```python
from build123d import *

# Parameters (mm, degrees)
SKETCH1_W           = 40.5
SKETCH1_H           = 37.5
PCB_DEPTH           = 1.64
FILLET1_R           = 2
MOUNT_HOLE_REACH    = 29.646
SKETCH2_R           = 1.45
SLOT_REACH          = 29.646
CUT_EXTRUDE3_REACH  = 29.646
SKETCH4_R           = 0.5
SKETCH5_W           = 34.6
SKETCH5_H           = 22.7
OLED_GLASS_DEPTH    = 1.6
SKETCH6_W           = 12
SKETCH6_H           = 3.8
BOSS_EXTRUDE3_DEPTH = 1
FILLET2_R           = 1


with BuildPart() as part:
    # Sketch1 → PCB (new body)
    with BuildSketch(Plane.XY):
        Rectangle(SKETCH1_W, SKETCH1_H)
    extrude(amount=PCB_DEPTH)

    # Fillet1
    fillet1_edges = [part.edges().sort_by_distance(p)[0] for p in [
        (-20.25, 18.75, 0.82),
        (20.25, 18.75, 0.82),
        (20.25, -18.75, 0.82),
        (-20.25, -18.75, 0.82),
    ]]
    fillet(fillet1_edges, radius=FILLET1_R)

    # Sketch2 → mount hole (cut, up to next)
    with BuildSketch(Plane.XY.offset(1.64), mode=Mode.PRIVATE) as mount_hole_sk1:
        with Locations((-17.75, 16.25)):
            Circle(SKETCH2_R)
    mount_hole_tool1 = extrude(mount_hole_sk1.sketch, amount=-MOUNT_HOLE_REACH, mode=Mode.PRIVATE) & part.part
    # Sketch2 → mount hole (cut, up to next)
    with BuildSketch(Plane.XY.offset(1.64), mode=Mode.PRIVATE) as mount_hole_sk2:
        with Locations((17.75, 16.25)):
            Circle(SKETCH2_R)
    mount_hole_tool2 = extrude(mount_hole_sk2.sketch, amount=-MOUNT_HOLE_REACH, mode=Mode.PRIVATE) & part.part
    # Sketch2 → mount hole (cut, up to next)
    with BuildSketch(Plane.XY.offset(1.64), mode=Mode.PRIVATE) as mount_hole_sk3:
        with Locations((17.75, -16.25)):
            Circle(SKETCH2_R)
    mount_hole_tool3 = extrude(mount_hole_sk3.sketch, amount=-MOUNT_HOLE_REACH, mode=Mode.PRIVATE) & part.part
    # Sketch2 → mount hole (cut, up to next)
    with BuildSketch(Plane.XY.offset(1.64), mode=Mode.PRIVATE) as mount_hole_sk4:
        with Locations((-17.75, -16.25)):
            Circle(SKETCH2_R)
    mount_hole_tool4 = extrude(mount_hole_sk4.sketch, amount=-MOUNT_HOLE_REACH, mode=Mode.PRIVATE) & part.part
    add(mount_hole_tool1.solids().sort_by_distance((-17.75, 16.25, 1.64))[0], mode=Mode.SUBTRACT)
    add(mount_hole_tool2.solids().sort_by_distance((17.75, 16.25, 1.64))[0], mode=Mode.SUBTRACT)
    add(mount_hole_tool3.solids().sort_by_distance((17.75, -16.25, 1.64))[0], mode=Mode.SUBTRACT)
    add(mount_hole_tool4.solids().sort_by_distance((-17.75, -16.25, 1.64))[0], mode=Mode.SUBTRACT)

    # Sketch3 → slot (cut, up to next)
    with BuildSketch(Plane.XY.offset(1.64), mode=Mode.PRIVATE) as slot_sk1:
        with BuildLine():
            Line((-9.4, -15.15), (9.4, -15.15))
            ThreePointArc((9.4, -15.15), (10, -15.75), (9.4, -16.35))
            Line((9.4, -16.35), (-9.4, -16.35))
            ThreePointArc((-9.4, -16.35), (-10, -15.75), (-9.4, -15.15))
        make_face()
    slot_tool1 = extrude(slot_sk1.sketch, amount=-SLOT_REACH, mode=Mode.PRIVATE) & part.part
    add(slot_tool1.solids().sort_by_distance((0, -15.75, 1.64))[0], mode=Mode.SUBTRACT)

    # Sketch4 → Cut-Extrude3 (cut, up to next)
    with BuildSketch(Plane.XY.offset(1.64), mode=Mode.PRIVATE) as cut_extrude3_sk1:
        with Locations((-8.89, 15.55)):
            Circle(SKETCH4_R)
    cut_extrude3_tool1 = extrude(cut_extrude3_sk1.sketch, amount=-CUT_EXTRUDE3_REACH, mode=Mode.PRIVATE) & part.part
    # Sketch4 → Cut-Extrude3 (cut, up to next)
    with BuildSketch(Plane.XY.offset(1.64), mode=Mode.PRIVATE) as cut_extrude3_sk2:
        with Locations((-6.35, 15.55)):
            Circle(SKETCH4_R)
    cut_extrude3_tool2 = extrude(cut_extrude3_sk2.sketch, amount=-CUT_EXTRUDE3_REACH, mode=Mode.PRIVATE) & part.part
    # Sketch4 → Cut-Extrude3 (cut, up to next)
    with BuildSketch(Plane.XY.offset(1.64), mode=Mode.PRIVATE) as cut_extrude3_sk3:
        with Locations((-3.81, 15.55)):
            Circle(SKETCH4_R)
    cut_extrude3_tool3 = extrude(cut_extrude3_sk3.sketch, amount=-CUT_EXTRUDE3_REACH, mode=Mode.PRIVATE) & part.part
    # Sketch4 → Cut-Extrude3 (cut, up to next)
    with BuildSketch(Plane.XY.offset(1.64), mode=Mode.PRIVATE) as cut_extrude3_sk4:
        with Locations((-1.27, 15.55)):
            Circle(SKETCH4_R)
    cut_extrude3_tool4 = extrude(cut_extrude3_sk4.sketch, amount=-CUT_EXTRUDE3_REACH, mode=Mode.PRIVATE) & part.part
    # Sketch4 → Cut-Extrude3 (cut, up to next)
    with BuildSketch(Plane.XY.offset(1.64), mode=Mode.PRIVATE) as cut_extrude3_sk5:
        with Locations((1.27, 15.55)):
            Circle(SKETCH4_R)
    cut_extrude3_tool5 = extrude(cut_extrude3_sk5.sketch, amount=-CUT_EXTRUDE3_REACH, mode=Mode.PRIVATE) & part.part
    # Sketch4 → Cut-Extrude3 (cut, up to next)
    with BuildSketch(Plane.XY.offset(1.64), mode=Mode.PRIVATE) as cut_extrude3_sk6:
        with Locations((3.81, 15.55)):
            Circle(SKETCH4_R)
    cut_extrude3_tool6 = extrude(cut_extrude3_sk6.sketch, amount=-CUT_EXTRUDE3_REACH, mode=Mode.PRIVATE) & part.part
    # Sketch4 → Cut-Extrude3 (cut, up to next)
    with BuildSketch(Plane.XY.offset(1.64), mode=Mode.PRIVATE) as cut_extrude3_sk7:
        with Locations((6.35, 15.55)):
            Circle(SKETCH4_R)
    cut_extrude3_tool7 = extrude(cut_extrude3_sk7.sketch, amount=-CUT_EXTRUDE3_REACH, mode=Mode.PRIVATE) & part.part
    # Sketch4 → Cut-Extrude3 (cut, up to next)
    with BuildSketch(Plane.XY.offset(1.64), mode=Mode.PRIVATE) as cut_extrude3_sk8:
        with Locations((8.89, 15.55)):
            Circle(SKETCH4_R)
    cut_extrude3_tool8 = extrude(cut_extrude3_sk8.sketch, amount=-CUT_EXTRUDE3_REACH, mode=Mode.PRIVATE) & part.part
    add(cut_extrude3_tool1.solids().sort_by_distance((-8.89, 15.55, 1.64))[0], mode=Mode.SUBTRACT)
    add(cut_extrude3_tool2.solids().sort_by_distance((-6.35, 15.55, 1.64))[0], mode=Mode.SUBTRACT)
    add(cut_extrude3_tool3.solids().sort_by_distance((-3.81, 15.55, 1.64))[0], mode=Mode.SUBTRACT)
    add(cut_extrude3_tool4.solids().sort_by_distance((-1.27, 15.55, 1.64))[0], mode=Mode.SUBTRACT)
    add(cut_extrude3_tool5.solids().sort_by_distance((1.27, 15.55, 1.64))[0], mode=Mode.SUBTRACT)
    add(cut_extrude3_tool6.solids().sort_by_distance((3.81, 15.55, 1.64))[0], mode=Mode.SUBTRACT)
    add(cut_extrude3_tool7.solids().sort_by_distance((6.35, 15.55, 1.64))[0], mode=Mode.SUBTRACT)
    add(cut_extrude3_tool8.solids().sort_by_distance((8.89, 15.55, 1.64))[0], mode=Mode.SUBTRACT)

    # Sketch5 → OLED glass (add)
    with BuildSketch(Plane.XY.offset(1.64)):
        with Locations((0, -0.6)):
            Rectangle(SKETCH5_W, SKETCH5_H)
    extrude(amount=OLED_GLASS_DEPTH)

    # Sketch6 → Boss-Extrude3 (add)
    with BuildSketch(Plane.XY.offset(1.64)):
        with Locations((0, -13.85)):
            Rectangle(SKETCH6_W, SKETCH6_H)
    extrude(amount=BOSS_EXTRUDE3_DEPTH)

    # Fillet2
    fillet2_edges = [part.edges().sort_by_distance(p)[0] for p in [
        (0, -15.75, 2.64),
    ]]
    fillet(fillet2_edges, radius=FILLET2_R - 0.0001)  # a hair under: the kernel refuses the full size


solid = part.part
```
Source: CAD feature listing. Evaluate the final solid. Frame: model axes, mm. A direction names the side the tool comes from. Coordinates: 2 decimals unless noted, no trailing zeros. Loops run counter-clockwise (first coordinate to the right, second up) from the corner with the lowest first, then second, coordinate; pieces in that order, holes last. Notation, with made-up numbers: (33, -32) -> (40, -32) arc R6 cw to (40, -23) -> close; hole circle Ø8 at (-30.75, -1). An arc over 180 degrees is marked (long way). One line per item, written item: value. Start each with the question number.
Q1. Section query B-B, the plane y = 6. Return the cut outline in (x, z), and give its area (3 significant figures).
Q2. Mould query, pull axis X, two halves, no side actions, for faces 1 (the face through (-19.68, -18.15, 0.83)), 2 (the face through (0, 18.75, 1)), 3 (the face through (19.65, -18.18, 0.83)), 4 (the face through (0, -16.35, 1)). Classes: pulls with the +X half, pulls with the -X half, needs draft (parallel to the pull), parting line crosses it, or undercut.
Q3. Line query: line 1 along Y through (x, z) = (1.27, 0.4); line 2 along X through (y, z) = (-15, 0.2); line 3 along X through (y, z) = (-15.5, 0.75). Output: solid intervals per line, ascending.
Q4. Section query C-C, the plane y = 15.55. Give the number of separate pieces and of enclosed holes in the cut face, and give its area (3 significant figures).
Q5. Contact query for flat-ended pins moving along their axis: P1, Ø4, axis at x = -17.75, y = 16.25, coming from the -Z side; P2, Ø4.5, axis at x = 17.75, y = 16.25, coming from the +Z side; P3, Ø1.3, axis at x = -8.5, z = 2.5, coming from the -Y side; P4, Ø2, axis at x = 1.5, y = -13.5, coming from the +Z side. Output: stop coordinate, or through.
Q6. Section query A-A, the plane x = 8.89. Return the cut outline in (y, z), and give its area (3 significant figures).
Q7. Set-up query: faces 5 (the face through (0, -13, 2.64)), 6 (the face through (-20.25, 0, 1)), 7 (the face through (17.3, -1, 2)), 8 (the face through (-10, -15.76, 0.83)). Return all of +Z, -Z, +X, -X, +Y, -Y with unobstructed straight access to the full face (end or side cutting, diameter ignored); none if empty.
Results:
1. outline: (-20.25, 0) -> (20.25, 0) -> (20.25, 1.64) -> (17.3, 1.64) -> (17.3, 3.24) -> (-17.3, 3.24) -> (-17.3, 1.64) -> (-20.25, 1.64) -> close
1. area: 122 mm^2
2. face 1: pulls with the -X half
2. face 2: needs draft
2. face 3: pulls with the +X half
2. face 4: undercut
3. line 1: -18.75 to -16.35, -15.15 to 15.05, 16.05 to 18.75
3. line 2: -20.25 to -18.48, -17.02 to 17.02, 18.48 to 20.25
3. line 3: -20.25 to -18.99, -16.51 to -9.95, 9.95 to 16.51, 18.99 to 20.25
4. separate pieces: 11
4. enclosed holes: 0
4. area: 45.0 mm^2
5. P1: z = 0
5. P2: z = 1.64
5. P3: y = -11.95
5. P4: z = 2.64
6. outline: (-18.75, 0) -> (-16.35, 0) -> (-16.35, 1.64) -> (-18.75, 1.64) -> close; (-15.15, 0) -> (15.05, 0) -> (15.05, 1.64) -> (10.75, 1.64) -> (10.75, 3.24) -> (-11.95, 3.24) -> (-11.95, 1.64) -> (-15.15, 1.64) -> close; (16.05, 0) -> (18.75, 0) -> (18.75, 1.64) -> (16.05, 1.64) -> close
6. area: 94.2 mm^2
7. face 5: +Z, +X, -X, -Y
7. face 6: +Z, -Z, -X, +Y, -Y
7. face 7: +Z, +X, +Y, -Y
7. face 8: +Z, -Z
